Autodesk Inventor part; units mm, degrees
ref_plane "YZ Plane" through (0, 0, 0) normal (1, 0, 0) x (0, 1, 0)
ref_plane "XZ Plane" through (0, 0, 0) normal (0, 1, 0) x (-1, 0, 0)
ref_plane "XY Plane" through (0, 0, 0) normal (0, 0, 1) x (1, 0, 0)
sketch "Sketch1" plane through (0, 0, 0) normal (1, 0, 0) x (0, 1, 0)
  circle A0 centre (0, 0) radius 10
  circle A1 centre (0, 0) radius 2.2
  dimension "d0" = 20
  dimension "d1" = 4.4
extrude "Extrusion1" add sketch "Sketch1" along normal blind 9
sketch "Sketch2" plane through (9, 0, 0) normal (1, 0, 0) x (0, 0, -1)
  circle A0 centre (0, 0) radius 5
  dimension "d4" = 10
extrude "Extrusion2" cut sketch "Sketch2" against normal blind 6
chamfer "Chamfer1" distance 1 distance2 9 1 edges at (9, -10, 0) measured on face at (9, 8.2243, -0.9986)
fillet "Fillet2" radius 1.5 2 edges at (9, -9.0005, 0) (9, 0, 5)
properties part number "rubberen_voetje" material "Rubber"
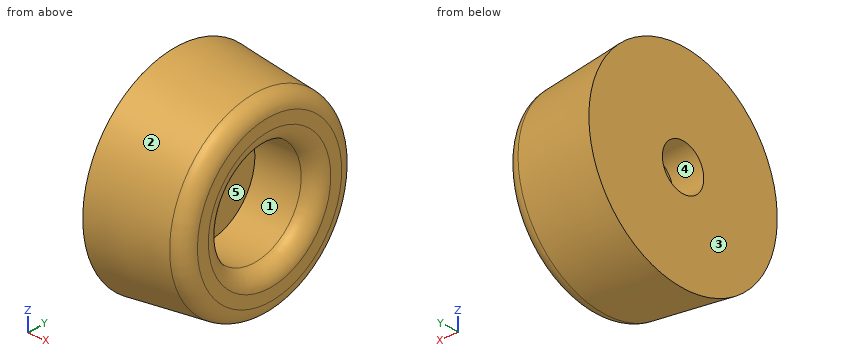
Input: part model. Units: mm. Frame: model coordinates. Face numbers are marked on the shaded views. A direction names the side the tool comes from. Give positions to 0.01 mm unless a question says otherwise; leave off trailing zeros. Write each loop counter-clockwise with the first axis right and the second up, starting at its lowest first coordinate (ties: lowest second). Pieces come first, ordered by that corner, then holes. Notation, with made-up numbers: (-21, 51.5) -> (26, 51.5) arc R8 cw to (26, 62.5) -> close; hole circle Ø8 at (-39, 58.25). An arc over 180 degrees is marked (long way). Use one line per item in the form item = value. Start each with the question number.
1) Draft query along Z for the marked faces 1, 2 and 3. Return one class per face: pulls with the +Z half, pulls with the -Z half, needs draft (parallel to the pull), parting line crosses it, or undercut.
2) Set-up query: the marked faces 4 and 5. Return all of +Z, -Z, +X, -X, +Y, -Y with unobstructed straight access to the full face (end or side cutting, diameter ignored); none if empty.
3) Section query C-C on x = 4.75. Return the cut outline in (y, z), then the cut area to 3 significant figures.
4) Pin query (flat end, axial travel): pin 1 (5 mm diameter, centred on x = 6, y = 0.5, fed in from -Z); pin 2 (2 mm diameter, centred on x = 1.5, z = 4, fed in from +Y); pin 3 (1 mm diameter, centred on x = 8, y = 3, fed in from -Z); pin 4 (6 mm diameter, centred on y = 0, z = 0, fed in from -X). Return the tip coordinate at first contact, or that it passes through.
5) Ray query, probe 1 along Z at (x, y) = (0.85, 0); probe 2 along Z at (x, y) = (1.9, 0); probe 3 along X at (y, z) = (-3.25, -2.75). Return the intervals inside material, ascending. Write a range as from..to.
6) Section query D-D on x = 2.25. Return the cut outline in (y, z).
Outcome:
q1.face_1 = undercut
q1.face_2 = parting line crosses it
q1.face_3 = needs draft
q2.face_4 = +X, -X
q2.face_5 = +X
q3.outline = circle Ø18.95 at (0, 0); hole circle Ø10 at (0, 0)
q3.area = 203 mm^2
q4.pin_1 = -9.61
q4.pin_2 = 9.39
q4.pin_3 = -8.77
q4.pin_4 = 0
q5.probe_1 = -9.91..-2.2, 2.2..9.91
q5.probe_2 = -9.79..-2.2, 2.2..9.79
q5.probe_3 = 0..3
q6.outline = circle Ø19.5 at (0, 0); hole circle Ø4.4 at (0, 0)
